The model under review builds one solid part; all positions refer to its coordinate system, in mm. Face numbers are marked on the shaded views. A direction names the side the tool comes from. Round coordinates to 2 decimals unless told otherwise and drop trailing zeros. Order: outer loops, then holes, each group sorted by start corner. A loop starts at its lowest first (then second) coordinate and runs counter-clockwise, first axis right, second up. Notation, with made-up numbers: M 69,73 L 109,73 A30 cw 109,104 Z; hole C -34,86.5 d6. An arc over 180 degrees is marked long. Use a Markdown table: item, result. Add a question column.
1. Consider section A-A on y = 8. State the section outline as (x, z) points.
2. To check wall thickness, follow probe 1 along X at (y, z) = (13.75, 7.25); probe 2 along Y at (x, z) = (-79, 3); probe 3 along Y at (x, z) = (-92.5, -1.25). State the ranges of each line that lie inside material, in increasing order.
3. Insertion check: P1, Ø8, axis at x = -27, z = -0.5, coming from the +Y side; P2, Ø5, axis at x = -90, z = 0.5, coming from the +Y side; P3, Ø10, axis at y = 5, z = -3, coming from the -X side; P4, Ø1, axis at x = -18.5, y = 4, coming from the -Z side. Each pin has a flat end and moves straight along its axis. Give the tip position at first contact, or say it passes through.
4. For the marked faces 1, 2 and 3, list the 3-axis set-ups (+Z, -Z, +X, -X, +Y, -Y) from which the entire face can be reached by the end or side of a thin tool; tool diameter is ignored.
5. Consider section B-B on z = 0. State the section outline as (x, y) points.
6. Consider section D-D on x = -115. State the section outline as (y, z) points, then the cut area to 3 significant figures.
7. Consider section C-C on x = -49.5. State the section outline as (y, z) points, then the cut area to 3 significant figures.
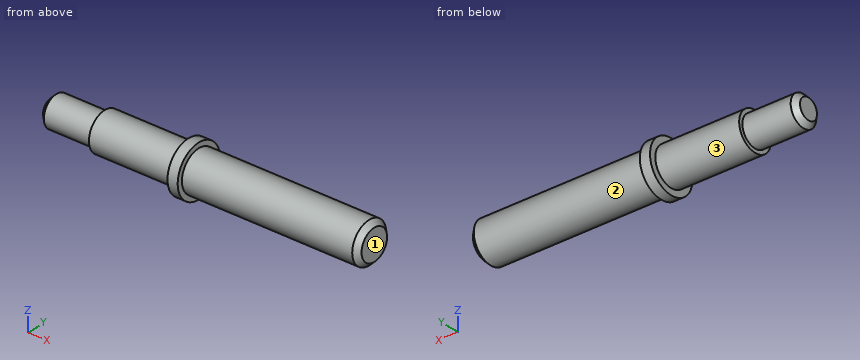
from build123d import *

# Parameters (mm, degrees)
SKIZZE2_R                       = 7.5
SKIZZE2_R_2                     = 6
SCHNITT_LINEAR_AUSTRAGEN2_DEPTH = 21
FASE2_SIZE                      = 2
FASE3_SIZE                      = 2


with BuildPart() as part:
    # Skizze1 → Rotation1 (revolve)
    with BuildSketch(Plane.XY):
        Polygon((0, 0), (-69, 0), (-69, -2), (-73, -2), (-73, 0.5), (-127, 0.5), (-127, 8), (0, 8), align=None)
    revolve(axis=Axis((-127, 8, 0), (1, 0, 0)))

    # Skizze2 → Schnitt-Linear austragen2 (cut)
    with BuildSketch(Plane.ZY.offset(127)):
        with Locations((0, 8)):
            Circle(SKIZZE2_R)
        with Locations((0, 8)):
            Circle(SKIZZE2_R_2, mode=Mode.SUBTRACT)
    extrude(amount=-SCHNITT_LINEAR_AUSTRAGEN2_DEPTH, mode=Mode.SUBTRACT)

    # Fase2
    fase2_edges = [part.edges().sort_by_distance(p)[0] for p in [
        (-127, 8, -6),
    ]]
    chamfer(fase2_edges, length=FASE2_SIZE)

    # Fase3
    fase3_edges = [part.edges().sort_by_distance(p)[0] for p in [
        (0, 16, 0),
    ]]
    chamfer(fase3_edges, length=FASE3_SIZE)


solid = part.part
Answer block:
| question | item | result |
|---|---|---|
| 1 | outline | M -127,-4 L -125,-6 L -106,-6 L -106,-7.5 L -73,-7.5 L -73,-10 L -69,-10 L -69,-8 L -2,-8 L 0,-6 L 0,6 L -2,8 L -69,8 L -69,10 L -73,10 L -73,7.5 L -106,7.5 L -106,6 L -125,6 L -127,4 Z |
| 2 | probe 1 | -73 to -69 |
| 2 | probe 2 | 1.13 to 14.87 |
| 2 | probe 3 | 0.6 to 15.4 |
| 3 | P1 | y = 16 |
| 3 | P2 | y = 15.5 |
| 3 | P3 | x = -127 |
| 3 | P4 | z = -7.19 |
| 4 | face 1 | +Z, -Z, +X, +Y, -Y |
| 4 | face 2 | +X |
| 4 | face 3 | -X |
| 5 | outline | M -127,4 L -125,2 L -106,2 L -106,0.5 L -73,0.5 L -73,-2 L -69,-2 L -69,0 L -2,0 L 0,2 L 0,14 L -2,16 L -69,16 L -69,18 L -73,18 L -73,15.5 L -106,15.5 L -106,14 L -125,14 L -127,12 Z |
| 6 | outline | C 8,0 d12 |
| 6 | area | 113 mm^2 |
| 7 | outline | C 8,0 d16 |
| 7 | area | 201 mm^2 |
